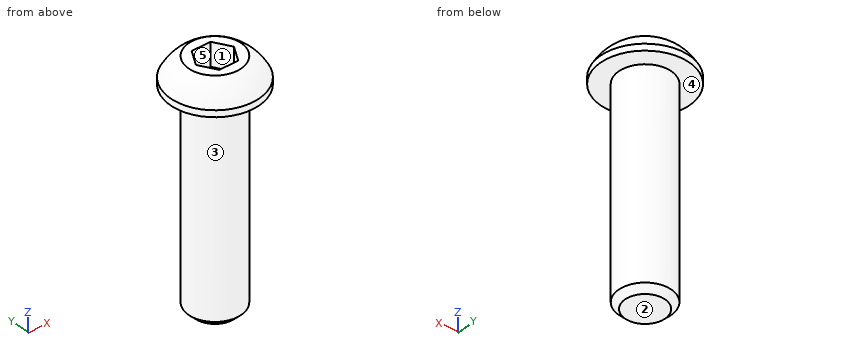
from build123d import *

# Parameters (mm, degrees)
F0_W     = 3.175
F0_H     = 25.4
F2_SIZE2 = 0.762
F2_SIZE  = 0.762
F4_DEPTH = 2.8194


with BuildPart() as f1:
    # F0 (on Front) → F1 (revolve)
    with BuildSketch(Plane.XZ):
        with Locations((1.5875, 12.7)):
            Rectangle(F0_W, F0_H)
        with BuildLine():
            Line((0, 28.575), (0, 25.4))
            Line((0, 25.4), (3.175, 25.4))
            Line((3.175, 25.4), (5.3594, 25.4))
            Line((5.3594, 25.4), (5.3594, 26.1874))
            ThreePointArc((5.3594, 26.1874), (4.431365, 27.531394), (3.175, 28.575))
            Line((3.175, 28.575), (0, 28.575))
        make_face()
    revolve(axis=Axis((0, 0, 12.7), (0, 0, 1)))

    # F2
    f2_edges = [f1.edges().sort_by_distance(p)[0] for p in [
        (-3.175, 0, 0),
    ]]
    chamfer(f2_edges, length=F2_SIZE, length2=F2_SIZE2)

    # F3 (on face) → F4 (cut)
    with BuildSketch(Plane.XY.offset(28.575)):
        Polygon((1.145679, 1.984375), (-1.145679, 1.984375), (-2.291359, 0), (-1.145679, -1.984375), (1.145679, -1.984375), (2.291359, 0), align=None)
    extrude(amount=-F4_DEPTH, mode=Mode.SUBTRACT)


solid = f1.part
Build history of the part. All positions in model axes, mm. Face numbers are marked on the shaded views. A direction names the side the tool comes from. Round coordinates to 2 decimals unless told otherwise and drop trailing zeros. Order: outer loops, then holes, each group sorted by start corner. A loop starts at its lowest first (then second) coordinate and runs counter-clockwise, first axis right, second up. Notation, with made-up numbers: M -19.75,-12.5 L -1.75,-12.5 A27 cw -1.75,23.5 Z; hole C 74.25,75 d5. An arc over 180 degrees is marked long. Use CSV: the item, a comma, the result in double quotes. Start each with the question number.
(1) Drill centre lines: probe 1 along Z at (x, y) = (-0.75, 1.5); probe 2 along Y at (x, z) = (-2.25, 5.25); probe 3 along Y at (x, z) = (0.5, 10). Where is each one in solid material? Low to high.
(2) Cut at A-A on z = 15.5. List the corners of the cut face in (x, y) (3 decimals), then the cut area to 3 significant figures.
(3) Mould opens along X. For the marked faces 3, 4 and 5 say: +X half, -X half, draft (parallel to the pull), parting line (faces both ways), or undercut.
(4) Tool access for the marked faces 1 and 2: list every direction of +Z, -Z, +X, -X, +Y, -Y with a clear straight run to the whole face (end or side of a thin tool).
(5) Flat gauge pins, fed straight in: P1, Ø1.2, axis at x = -1, y = -0.5, coming from the +Z side; P2, Ø1, axis at x = 4, y = 0, coming from the -Z side; P3, Ø4, axis at y = -3, z = 11, coming from the -X side; P4, Ø1.1, axis at x = 0.5, z = 26.5, coming from the -Y side. Where does each tip first touch, or does it go through?
Findings:
1,probe 1,"z = 0 to 25.76"
1,probe 2,"y = -2.24 to 2.24"
1,probe 3,"y = -3.14 to 3.14"
2,outline,"C 0,0 d6.35"
2,area,"31.7 mm^2"
3,face 3,"parting line"
3,face 4,"draft"
3,face 5,"undercut"
4,face 1,"+Z"
4,face 2,"-Z, +X, -X, +Y, -Y"
5,P1,"stops at z = 25.76"
5,P2,"stops at z = 25.4"
5,P3,"stops at x = -3.01"
5,P4,"stops at y = -5.36"
